The model under review builds one solid part; all positions refer to its coordinate system, in mm. Round coordinates to 2 decimals unless told otherwise and drop trailing zeros. Order: outer loops, then holes, each group sorted by start corner. A loop starts at its lowest first (then second) coordinate and runs counter-clockwise, first axis right, second up. Notation, with made-up numbers: M 65.25,29.25 L 79.25,29.25 A19 cw 79.25,50.25 Z; hole C -5,28.5 d4. An arc over 180 degrees is marked long. Answer as a JSON object with one key per item and string values. Group by question number.
1) Insertion check: pin 1 Ø4 at (x, y) = (-7, -8.5) entering from -Z; pin 2 Ø12 at (x, y) = (-13, -7) entering from +Z; pin 3 Ø12 at (x, y) = (-27, -23) entering from +Z. Each pin has a flat end and moves straight along its axis. Give the tip position at first contact, or say it passes through.
2) Consider section C-C, the plane z = 13. Write out the cut boundary in (x, y), then the cut area to 3 significant figures.
3) Consider section B-B, the plane x = -10. Write out the cut boundary in (y, z).
4) To check wall thickness, follow line 1 (Z direction, x = -8, y = -13); line 2 (Z direction, x = -39, y = -27). State the ranges of each line that lie inside material, in increasing order.
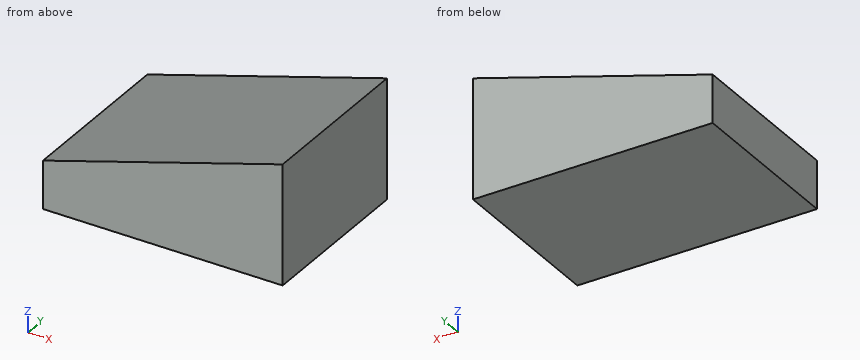
```python
from build123d import *

# Parameters (mm, degrees)
F0_W     = 50
F0_H     = 25
F1_DEPTH = 35
F2_SIZE2 = 49.99999
F2_SIZE  = 14.99999


# Not quite as in the source:
# - a fillet or chamfer is up to 0.001 mm smaller than in the source, because OpenCascade refuses the exact size


with BuildPart() as f1:
    # F0 (on Front) → F1 (new body)
    with BuildSketch(Plane.XZ):
        with Locations((-25, 12.5)):
            Rectangle(F0_W, F0_H)
    extrude(amount=F1_DEPTH)

    # F2 (size 15 and 50 in the source; OpenCascade refuses exactly that, so slightly less here)
    f2_edges = [f1.edges().sort_by_distance(p)[0] for p in [
        (-50, -17.5, 25),
    ]]
    f2_side = f1.faces().sort_by_distance((-50, -17.5, 12.5))[0]
    chamfer(f2_edges, length=F2_SIZE, length2=F2_SIZE2, reference=f2_side)


solid = f1.part
```
Results list:
{
 "1": {"pin 1": "z = 0", "pin 2": "z = 22.9", "pin 3": "z = 18.7"},
 "2": {"outline": "M -40,-35 L 0,-35 L 0,0 L -40,0 Z", "area": "1,400 mm^2"},
 "3": {"outline": "M -35,0 L 0,0 L 0,22 L -35,22 Z"},
 "4": {"line 1": "0 to 22.6", "line 2": "0 to 13.3"}
}
